Geometry check sheet. Reference: drawing and pictorial views, mm from the part's lowest x, y, z. Coordinates: 2 decimals unless noted, no trailing zeros. Order: outer loops, then holes, each group sorted by start corner. A loop starts at its lowest first (then second) coordinate and runs counter-clockwise, first axis right, second up. Notation, with made-up numbers: M 68.25,65.5 L 111.25,65.5 A25 ccw 111.25,87.5 Z; hole C -39,0.5 d8. An arc over 180 degrees is marked long. Return JSON: item names as keys, results as strings.
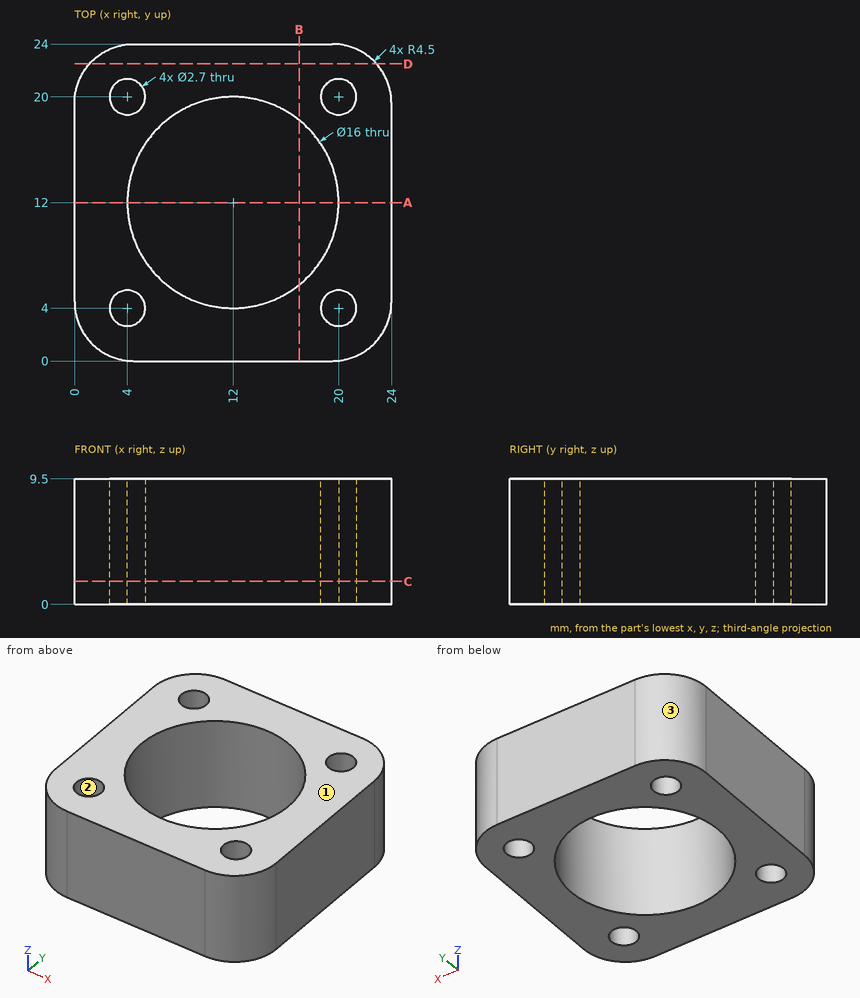
Q1. Cross-section at A-A, the plane y = 12. Record the boundary of the cut face in (x, z), and give its area (3 significant figures).
Values:
{"outline": "M 0,0 L 4,0 L 4,9.5 L 0,9.5 Z; M 20,0 L 24,0 L 24,9.5 L 20,9.5 Z", "area": "76.0 mm^2"}
Q2. Cross-section at C-C, the plane z = 1.75. Record the boundary of the cut face in (x, y).
Values:
{"outline": "M 0,4.5 A4.5 ccw 4.5,0 L 19.5,0 A4.5 ccw 24,4.5 L 24,19.5 A4.5 ccw 19.5,24 L 4.5,24 A4.5 ccw 0,19.5 Z; hole C 4,4 d2.7; hole C 4,20 d2.7; hole C 12,12 d16; hole C 20,4 d2.7; hole C 20,20 d2.7"}
Q3. Draft check along Y on the marked faces 1, 2 and 3. Enter one of: pulls with the +Y half, pulls with the -Y half, needs draft (parallel to the pull), parting line crosses it, or undercut.
Values:
{"face 1": "needs draft", "face 2": "undercut", "face 3": "pulls with the +Y half"}
Q4. Cross-section at D-D, the plane y = 22.5. Record the boundary of the cut face in (x, z), and give its area (3 significant figures).
Values:
{"outline": "M 1.15,0 L 22.85,0 L 22.85,9.5 L 1.15,9.5 Z", "area": "206 mm^2"}
Q5. Cross-section at B-B, the plane x = 17. Record the boundary of the cut face in (y, z) (3 decimals), and give its area (3 significant figures).
Values:
{"outline": "M 0,0 L 5.755,0 L 5.755,9.5 L 0,9.5 Z; M 18.245,0 L 24,0 L 24,9.5 L 18.245,9.5 Z", "area": "109 mm^2"}
Q6. Material ranges on line 1 along X through (y, z) = (5, 7.5); line 2 along X through (y, z) = (21, 6.75); line 3 along Y through (x, z) = (12, 5), recorded low to high.
Values:
{"line 1": "0 to 3.09, 4.91 to 8.13, 15.87 to 19.09, 20.91 to 24", "line 2": "0.26 to 3.09, 4.91 to 19.09, 20.91 to 23.74", "line 3": "0 to 4, 20 to 24"}
Q7. Go/stop test with a flat-tipped pin: pin 1 (9.5 mm diameter, centred on x = 12, y = 12, fed in from -Z). Record where the tip stops, or that it passes through.
Values:
{"pin 1": "through"}
